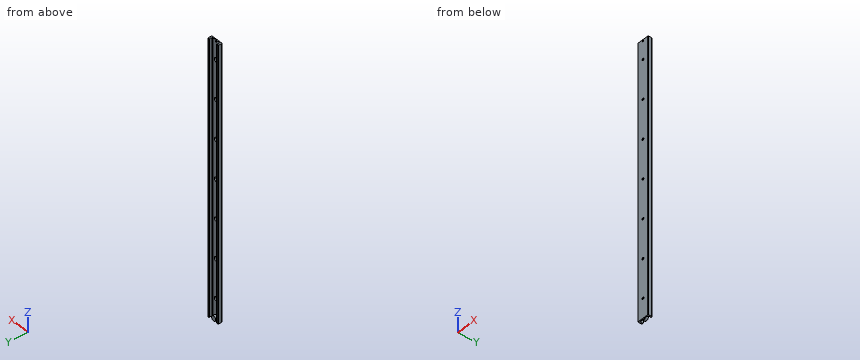
```python
from build123d import *

# Parameters (mm, degrees)
EXTRUDE_1_DEPTH          = 720
SKETCH_3_R               = 5
EXTRUDE_3_DEPTH          = 5
HOLE_WIZARD_1_AT_2_COUNT = 2
HOLE_WIZARD_1_AT_2_PITCH = 640
HOLE_WIZARD_1_AT_3_COUNT = 2
HOLE_WIZARD_1_AT_3_PITCH = 560
HOLE_WIZARD_1_AT_4_COUNT = 2
HOLE_WIZARD_1_AT_4_PITCH = 480
HOLE_WIZARD_1_AT_5_COUNT = 2
HOLE_WIZARD_1_AT_5_PITCH = 400
HOLE_WIZARD_1_AT_6_COUNT = 2
HOLE_WIZARD_1_AT_6_PITCH = 320
HOLE_WIZARD_1_AT_7_COUNT = 2
HOLE_WIZARD_1_AT_7_PITCH = 240
HOLE_WIZARD_1_AT_8_COUNT = 2
HOLE_WIZARD_1_AT_8_PITCH = 160
HOLE_WIZARD_1_AT_9_COUNT = 2
HOLE_WIZARD_1_AT_9_PITCH = 80
FILLET_1_R               = 0.5
FILLET_2_R               = 1
SKETCH_6_W               = 28.389485075
SKETCH_6_H               = 8.5
CUT_EXTRUDE_1_DEPTH      = 160
SKETCH_7_R               = 1.5
CUT_EXTRUDE_2_DEPTH      = 561.177204106


with BuildPart() as part:
    # ｽｹｯﾁ1 → ﾎﾞｽ - 押し出し1 (new body)
    with BuildSketch(Plane.XY.offset(720)):
        with BuildLine():
            Line((8.5, 3.408712153), (8.5, 2))
            Line((8.5, 2), (-8.5, 2))
            Line((-8.5, 2), (-8.5, 3.408712153))
            ThreePointArc((-8.5, 3.408712153), (-9.999347871, 5.642901666), (-8.603592403, 7.943230663))
            ThreePointArc((-8.603592403, 7.943230663), (-8.97237829, 8.349479447), (-9.5, 8.5))
            Line((-9.5, 8.5), (-12.5, 8.5))
            Line((-12.5, 8.5), (-12.5, 0))
            Line((-12.5, 0), (12.5, 0))
            Line((12.5, 0), (12.5, 8.5))
            Line((12.5, 8.5), (9.5, 8.5))
            ThreePointArc((9.5, 8.5), (8.97237829, 8.349479447), (8.603592403, 7.943230663))
            ThreePointArc((8.603592403, 7.943230663), (9.999347871, 5.642901666), (8.5, 3.408712153))
        make_face()
    extrude(amount=-EXTRUDE_1_DEPTH)

    # ｽｹｯﾁ3 → ﾎﾞｽ - 押し出し3 (add)
    with BuildSketch(Plane(origin=(0, 2, 0), x_dir=(-1, 0, 0), z_dir=(0, 1, 0))):
        with Locations(Location((0, 3, 0), (0, 0, 323.130102354))):
            Circle(SKETCH_3_R)
    extrude(amount=EXTRUDE_3_DEPTH)

    # ｽｹｯﾁ4 → 穴1 (revolve, cut)
    with BuildSketch(Plane(origin=(0, 2, 40), x_dir=(0, 0, 1), z_dir=(1, 0, 0))):
        Polygon((0, 0), (0, 2), (2.25, 2), (4.25, 0), align=None)
    hole_wizard_1 = revolve(axis=Axis((0, -108, 40), (0, 1, 0)), mode=Mode.SUBTRACT)

    # 穴1 at 2: 穴1 ×2
    with Locations(*[(0, 0, i * HOLE_WIZARD_1_AT_2_PITCH) for i in range(1, HOLE_WIZARD_1_AT_2_COUNT)]):
        add(hole_wizard_1, mode=Mode.SUBTRACT)

    # 穴1 at 3: 穴1 ×2
    with Locations(*[(0, 0, i * HOLE_WIZARD_1_AT_3_PITCH) for i in range(1, HOLE_WIZARD_1_AT_3_COUNT)]):
        add(hole_wizard_1, mode=Mode.SUBTRACT)

    # 穴1 at 4: 穴1 ×2
    with Locations(*[(0, 0, i * HOLE_WIZARD_1_AT_4_PITCH) for i in range(1, HOLE_WIZARD_1_AT_4_COUNT)]):
        add(hole_wizard_1, mode=Mode.SUBTRACT)

    # 穴1 at 5: 穴1 ×2
    with Locations(*[(0, 0, i * HOLE_WIZARD_1_AT_5_PITCH) for i in range(1, HOLE_WIZARD_1_AT_5_COUNT)]):
        add(hole_wizard_1, mode=Mode.SUBTRACT)

    # 穴1 at 6: 穴1 ×2
    with Locations(*[(0, 0, i * HOLE_WIZARD_1_AT_6_PITCH) for i in range(1, HOLE_WIZARD_1_AT_6_COUNT)]):
        add(hole_wizard_1, mode=Mode.SUBTRACT)

    # 穴1 at 7: 穴1 ×2
    with Locations(*[(0, 0, i * HOLE_WIZARD_1_AT_7_PITCH) for i in range(1, HOLE_WIZARD_1_AT_7_COUNT)]):
        add(hole_wizard_1, mode=Mode.SUBTRACT)

    # 穴1 at 8: 穴1 ×2
    with Locations(*[(0, 0, i * HOLE_WIZARD_1_AT_8_PITCH) for i in range(1, HOLE_WIZARD_1_AT_8_COUNT)]):
        add(hole_wizard_1, mode=Mode.SUBTRACT)

    # 穴1 at 9: 穴1 ×2
    with Locations(*[(0, 0, i * HOLE_WIZARD_1_AT_9_PITCH) for i in range(1, HOLE_WIZARD_1_AT_9_COUNT)]):
        add(hole_wizard_1, mode=Mode.SUBTRACT)

    # ﾌｨﾚｯﾄ1
    fillet_1_edges = [part.edges().sort_by_distance(p)[0] for p in [
        (-8.5, 2, 360),
        (8.5, 2, 360),
    ]]
    fillet(fillet_1_edges, radius=FILLET_1_R)

    # ﾌｨﾚｯﾄ2
    fillet_2_edges = [part.edges().sort_by_distance(p)[0] for p in [
        (12.5, 8.5, 360),
        (12.5, 0, 360),
        (-12.5, 0, 360),
        (-12.5, 8.5, 360),
    ]]
    fillet(fillet_2_edges, radius=FILLET_2_R)

    # ｽｹｯﾁ6 → ｶｯﾄ - 押し出し1 (cut)
    with BuildSketch(Plane.XY.offset(720)):
        with Locations((-0.090556571, 4.25)):
            Rectangle(SKETCH_6_W, SKETCH_6_H)
    extrude(amount=-CUT_EXTRUDE_1_DEPTH, mode=Mode.SUBTRACT)

    # ｽｹｯﾁ7 → ｶｯﾄ - 押し出し2 (cut, through all)
    with BuildSketch(Plane(origin=(0, 2, 0), x_dir=(1, 0, 0), z_dir=(0, 1, 0))):
        with Locations(Location((0, -557, 0), (0, 0, 270))):
            Circle(SKETCH_7_R)
    extrude(amount=-CUT_EXTRUDE_2_DEPTH, mode=Mode.SUBTRACT)


solid = part.part
```
Source: CAD feature listing. Evaluate the final solid. Frame: model axes, mm. Round coordinates to 2 decimals unless told otherwise and drop trailing zeros. Loops run counter-clockwise (first coordinate to the right, second up) from the corner with the lowest first, then second, coordinate; pieces in that order, holes last.
(1) Contact query for flat-ended pins moving along their axis: pin 1 Ø3.5 at (x, z) = (0, 557) entering from +Y; pin 2 Ø8 at (x, z) = (0.5, 2) entering from +Y; pin 3 Ø3 at (x, z) = (-7.5, 97.5) entering from +Y. Output: stop coordinate, or through.
From the geometry:
pin 1: stops at y = 2
pin 2: stops at y = 7
pin 3: stops at y = 8.37
(2) Material intervals for probe 1 along X at (y, z) = (3, 450.5); probe 2 along X at (y, z) = (6.25, 486.5); probe 3 along Y at (x, z) = (-7.25, 461), sorted ascending.
From the geometry:
probe 1: x = -12.5 to -8.5, 8.5 to 12.5
probe 2: x = -12.5 to -9.94, 9.94 to 12.5
probe 3: y = 0 to 2
(3) Section query A-A (z = 189). Output: boundary loops of the cut face in (x, y).
From the geometry:
outline: (-12.5, 1) arc R1 ccw to (-11.5, 0) - (11.5, 0) arc R1 ccw to (12.5, 1) - (12.5, 7.5) arc R1 ccw to (11.5, 8.5) - (9.5, 8.5) arc R1 ccw to (8.6, 7.94) arc R2.5 cw to (8.5, 3.41) - (8.5, 2.5) arc R0.5 cw to (8, 2) - (-8, 2) arc R0.5 cw to (-8.5, 2.5) - (-8.5, 3.41) arc R2.5 cw to (-8.6, 7.94) arc R1 ccw to (-9.5, 8.5) - (-11.5, 8.5) arc R1 ccw to (-12.5, 7.5) - close
